Build history of the part. All positions in model axes, mm. A direction names the side the tool comes from. Round coordinates to 2 decimals unless told otherwise and drop trailing zeros. Write each loop counter-clockwise with the first axis right and the second up, starting at its lowest first coordinate (ties: lowest second). Pieces come first, ordered by that corner, then holes.
Item 1: Band-saw the part on D-D, the plane y = 10.5. Write the cut outline in (x, z), then the cut area to 3 significant figures.
Item 2: 3-axis set-ups, long thin cutter, end or side, ignore diameter. For faces 1 (the cylindrical face through (0, 11, 3)), 2 (the flat face through (-3, 0, 6)): which of +Z, -Z, +X, -X, +Y, -Y reach the whole face in a straight line?
Item 3: Band-saw the part on B-B, the plane x = 5.75. Write the cut outline in (y, z), then the cut area to 3 significant figures.
Item 4: Wall check: probe 1 along Y at (x, z) = (0, 0.55); probe 2 along Y at (x, z) = (8.5, 3.55); probe 3 along X at (y, z) = (-3.25, 5.4). Give the ranges that are in metal, low to high.
Item 5: Band-saw the part on C-C, the plane z = 5.3. Write the cut outline in (x, y).
Item 6: Band-saw the part on A-A, the plane y = -10. Write the cut outline in (x, z), then the cut area to 3 significant figures.
Item 7: Drop flat-ended pins along their axis: pin 1 Ø1 at (y, z) = (1, 2) entering from -X; pin 2 Ø1.2 at (y, z) = (-1, 3.5) entering from +X; pin 3 Ø3 at (x, z) = (7, 4.5) entering from -Y (3 decimals). Give the stop position or say it passes through.
Item 8: Mould opens along X. For faces 3 (the flat face through (-3, 0, 0)), 4 (the cylindrical face through (-8.15, 3.6, 3.04)) say: +X half, -X half, draft (parallel to the pull), parting line (faces both ways), or undercut.
```python
from build123d import *
from build123d.topology import SkipClean

# Parameters (mm, degrees)
BOSS_EXTRUDE1_DEPTH = 6
CUT_EXTRUDE1_DEPTH  = 6


with BuildPart() as part:
    # Sketch1 → Boss-Extrude1 (new body)
    with BuildSketch(Plane.XY):
        with BuildLine():
            Line((1.5, 2), (1.5, 0))
            Line((1.5, 0), (7.5, 0))
            ThreePointArc((7.5, 0), (9, 1.5), (10.5, 0))
            Line((10.5, 0), (12.5, 0))
            ThreePointArc((12.5, 0), (8.838834765, 8.838834765), (0, 12.5))
            Line((0, 12.5), (0, 2.5))
            ThreePointArc((0, 2.5), (0.790569415, 2.371708245), (1.5, 2))
        make_face()
    extrude(amount=BOSS_EXTRUDE1_DEPTH)

    # Mirror4: part across plane


with BuildPart() as part_1:
    add(part.part)
    add(part.part.mirror(Plane(origin=(0, 12.5, 6), x_dir=(0, 0, 1), z_dir=(1, 0, 0))))

    # Sketch2 → Cut-Extrude1 (cut)
    with BuildSketch(Plane.XY.offset(6)):
        with BuildLine():
            ThreePointArc((8.411764706, 7.088174274), (0, 11), (-8.411764706, 7.088174274))
            ThreePointArc((-8.411764706, 7.088174274), (-8.110948699, 3.565460869), (-4.588235294, 3.866276877))
            ThreePointArc((-4.588235294, 3.866276877), (0, 6), (4.588235294, 3.866276877))
            ThreePointArc((4.588235294, 3.866276877), (8.110948699, 3.565460869), (8.411764706, 7.088174274))
        make_face()
    extrude(amount=-CUT_EXTRUDE1_DEPTH, mode=Mode.SUBTRACT)

    # Mirror5: part across plane


with BuildPart() as part_2:
    with SkipClean():  # the faces are left unmerged after this step: merging them gives an invalid solid
        add(part_1.part)
        add(part_1.part.mirror(Plane(origin=(-1.5, 0, 6), x_dir=(0, 0, 1), z_dir=(0, 1, 0))))


solid = part_2.part
```
Results:
1. outline: (-6.78, 0) - (-3.28, 0) - (-3.28, 6) - (-6.78, 6) - close; (3.28, 0) - (6.78, 0) - (6.78, 6) - (3.28, 6) - close
1. area: 42.0 mm2
2. face 1: +Z, -Z
2. face 2: +Z, +X, -X, +Y, -Y
3. outline: (-11.1, 0) - (-9.38, 0) - (-9.38, 6) - (-11.1, 6) - close; (-3.09, 0) - (3.09, 0) - (3.09, 6) - (-3.09, 6) - close; (9.38, 0) - (11.1, 0) - (11.1, 6) - (9.38, 6) - close
3. area: 57.8 mm2
4. probe 1: y = -12.5 to -11, -6 to -2.5, 2.5 to 6, 11 to 12.5
4. probe 2: y = -9.17 to -6.98, -3.98 to -1.41, 1.41 to 3.98, 6.98 to 9.17
4. probe 3: x = -12.07 to -7.64, -5.36 to 5.36, 7.64 to 12.07
5. outline: circle Ø25 at (0, 0); hole circle Ø3 at (-9, 0); hole (-8.41, -7.09) arc R11 ccw to (8.41, -7.09) arc R2.5 ccw to (4.59, -3.87) arc R6 cw to (-4.59, -3.87) arc R2.5 ccw to start; hole (-8.41, 7.09) arc R2.5 ccw to (-4.59, 3.87) arc R6 cw to (4.59, 3.87) arc R2.5 ccw to (8.41, 7.09) arc R11 ccw to start; hole (-1.5, -2) arc R2.5 ccw to (1.5, -2) - (1.5, 2) arc R2.5 ccw to (-1.5, 2) - close; hole circle Ø3 at (9, 0)
6. outline: (-7.5, 0) - (-4.58, 0) - (-4.58, 6) - (-7.5, 6) - close; (4.58, 0) - (7.5, 0) - (7.5, 6) - (4.58, 6) - close
6. area: 35.0 mm2
7. pin 1: stops at x = -12.49
7. pin 2: stops at x = 12.49
7. pin 3: stops at y = -11.225
8. face 3: draft
8. face 4: undercut
